Read the model definition and answer for the solid it produces. Units are mm, in the model's axes. Coordinates: 2 decimals unless noted, no trailing zeros. Write each loop counter-clockwise with the first axis right and the second up, starting at its lowest first coordinate (ties: lowest second). Pieces come first, ordered by that corner, then holes. Notation, with made-up numbers: (68.25, -32.5) -> (116.25, -32.5) arc R12 cw to (116.25, -28.5) -> close; hole circle Ø3 at (-23, 32). An arc over 180 degrees is marked (long way). Answer in a Markdown table with one row per item. Add a question column.
Item 1: For a pull along Y with two mould halves and no side action, classify faces 1 (the face through (-66.018, -51.804, 12.522)), 2 (the face through (-55, -47, 25.4)), 3 (the face through (-91.587, -28.426, 12.522)) as +Y half, -Y half, draft (parallel to the pull), parting line (faces both ways), or undercut.
Item 2: Straight lines are drawn through the part: line 1 (X direction, y = -1.5, z = 22.5); line 2 (Y direction, x = -71, z = 23.25); line 3 (X direction, y = -39, z = 18). For each, find the intervals that lie inside material, in ascending order. Write a range as from..to.
Item 3: Section B-B on x = -69.5 is taken. Write down the section's boundary in (y, z), then the cut area to 3 significant figures.
Item 4: Section A-A on y = 0 is taken. Write down the section's boundary in (x, z).
Item 5: Section C-C on z = 6 is taken. Write down the section's boundary in (x, y).
Item 6: Given pin 1 Ø8 at (x, z) = (-87.5, 4.5) entering from +Y; pin 2 Ø1.5 at (x, z) = (-50, 18) entering from +Y; pin 3 Ø2 at (y, z) = (-38, 7.5) entering from +X, each flat-ended and moving along its own axis, determine where each tip first touches the part or whether it passes through.
```python
from build123d import *

# Parameters (mm, degrees)
F0_R     = 53.853392601
F2_DEPTH = 25.4
F1_R     = 53.065742398
F4_T     = -6.35


with BuildPart() as f2:
    # F0 (on Top) → F2 (new body)
    with BuildSketch(Plane.XY):
        with Locations((-53.853392601, 0)):
            Circle(F0_R)
    extrude(amount=F2_DEPTH)


with BuildPart() as f2b:
    # F1 (on Top) → F2, piece 2 (new body)
    with BuildSketch(Plane.XY):
        with Locations((-54.5146726072, 0)):
            Circle(F1_R)
    extrude(amount=F2_DEPTH)

    # F4
    f4_openings = [f2b.faces().sort_by_distance(p)[0] for p in [
        (-54.514673, 0, 0),
        (-54.514673, 0, 25.4),
    ]]
    offset(amount=F4_T, openings=f4_openings)


solid = f2b.part
```
Results below:
| question | item | result |
|---|---|---|
| 1 | face 1 | parting line |
| 1 | face 2 | draft |
| 1 | face 3 | undercut |
| 2 | line 1 | x = -107.56..-101.21, -7.82..-1.47 |
| 2 | line 2 | y = -50.44..-43.71, 43.71..50.44 |
| 2 | line 3 | x = -90.5..-80.23, -28.8..-18.53 |
| 3 | outline | (-50.91, 0) -> (-44.25, 0) -> (-44.25, 25.4) -> (-50.91, 25.4) -> close; (44.25, 0) -> (50.91, 0) -> (50.91, 25.4) -> (44.25, 25.4) -> close |
| 3 | area | 338 mm2 |
| 4 | outline | (-107.58, 0) -> (-101.23, 0) -> (-101.23, 25.4) -> (-107.58, 25.4) -> close; (-7.8, 0) -> (-1.45, 0) -> (-1.45, 25.4) -> (-7.8, 25.4) -> close |
| 5 | outline | circle Ø106.13 at (-54.51, 0); hole circle Ø93.43 at (-54.51, 0) |
| 6 | pin 1 | stops at y = 44.45 |
| 6 | pin 2 | stops at y = 52.93 |
| 6 | pin 3 | stops at x = -16.48 |
